Here's how the part is built. I have some questions about the finished solid (model axes, mm). A direction names the side the tool comes from. Coordinates: 2 decimals unless noted, no trailing zeros. Write each loop counter-clockwise with the first axis right and the second up, starting at its lowest first coordinate (ties: lowest second). Pieces come first, ordered by that corner, then holes.
Item 1: I want a section at B-B (y = -24). Please give me the cut outline in (x, z).
Item 2: I'm going to push flat-ended pins straight in: P1, Ø1.7, axis at y = 34, z = 107, coming from the +X side; P2, Ø1.8, axis at x = 4.5, y = 14, coming from the +Z side; P3, Ø1.8, axis at x = 4.5, z = 65.5, coming from the +Y side; P4, Ø3, axis at x = 3.5, y = -121.5, coming from the -Z side. Where does each tip first touch, or does it pass through?
Item 3: I want a section at C-C (x = 4). Count the separate pieces of the cut face and the enclosed holes in it, and give its area (3 significant figures).
Item 4: I want a section at A-A (z = -20.5). Please give me the cut outline in (x, y).
Item 5: For faces 1 (the face through (3, 59, 104)), 2 (the face through (3, 122, 80)), 3 (the face through (3, -59, -104)), which set-ups out of +Z, -Z, +X, -X, +Y, -Y let a thin tool reach every point of the face, with its end or its side?
Item 6: Please list where these lines run through material, in increasing order: line 1 (Y direction, x = 3.2, z = -45); line 2 (Y direction, x = 5.05, z = -76.5); line 3 (Z direction, x = 2.2, y = -13).
Item 7: If we mould it in two halves opening along Z, with no side actions, what happens to faces 4 (the face through (3, 125, -85)), 5 (the face through (3, -122, -80)), 6 (the face through (3, -104, 104))? For each: pulls with the +Z half, pulls with the -Z half, needs draft (parallel to the pull), parting line crosses it, or undercut.
from build123d import *

# Parameters (mm, degrees)
ESQUISSE1_W             = 208
ESQUISSE1_H             = 238
BOSS_EXTRU_1_DEPTH      = 6
ESQUISSE3_W             = 10
ESQUISSE3_H             = 6
ESQUISSE3_W_2           = 6
ESQUISSE3_H_2           = 10
BOSS_EXTRU_5_DEPTH      = 6
ESQUISSE4_R             = 1.4
ENL_V_MAT_EXTRU_1_DEPTH = 6


with BuildPart() as part:
    # Esquisse1 → Boss.-Extru.1 (new body)
    with BuildSketch(Plane(origin=(0, 0, 0), x_dir=(0, 0, -1), z_dir=(1, 0, 0))):
        Rectangle(ESQUISSE1_W, ESQUISSE1_H)
    extrude(amount=BOSS_EXTRU_1_DEPTH)

    # Esquisse3 → Boss.-Extru.5 (add)
    with BuildSketch(Plane(origin=(6, 0, 0), x_dir=(0, 0, -1), z_dir=(1, 0, 0))):
        with Locations((-85, -122)):
            Rectangle(ESQUISSE3_W, ESQUISSE3_H)
        with Locations((-45, -122)):
            Rectangle(ESQUISSE3_W, ESQUISSE3_H)
        with Locations((107, -34)):
            Rectangle(ESQUISSE3_W_2, ESQUISSE3_H_2)
        with Locations((-107, -84)):
            Rectangle(ESQUISSE3_W_2, ESQUISSE3_H_2)
        with Locations((-107, -34)):
            Rectangle(ESQUISSE3_W_2, ESQUISSE3_H_2)
        with Locations((107, -84)):
            Rectangle(ESQUISSE3_W_2, ESQUISSE3_H_2)
        with Locations((45, -122)):
            Rectangle(ESQUISSE3_W, ESQUISSE3_H)
        with Locations((85, -122)):
            Rectangle(ESQUISSE3_W, ESQUISSE3_H)
        with Locations((85, 122)):
            Rectangle(ESQUISSE3_W, ESQUISSE3_H)
        with Locations((45, 122)):
            Rectangle(ESQUISSE3_W, ESQUISSE3_H)
        with Locations((107, 84)):
            Rectangle(ESQUISSE3_W_2, ESQUISSE3_H_2)
        with Locations((107, 34)):
            Rectangle(ESQUISSE3_W_2, ESQUISSE3_H_2)
        with Locations((-107, 34)):
            Rectangle(ESQUISSE3_W_2, ESQUISSE3_H_2)
        with Locations((-107, 84)):
            Rectangle(ESQUISSE3_W_2, ESQUISSE3_H_2)
        with Locations((-45, 122)):
            Rectangle(ESQUISSE3_W, ESQUISSE3_H)
        with Locations((-85, 122)):
            Rectangle(ESQUISSE3_W, ESQUISSE3_H)
    extrude(amount=-BOSS_EXTRU_5_DEPTH)

    # Esquisse4 → Enlèv. mat.-Extru.1 (cut)
    with BuildSketch(Plane(origin=(6, 0, 0), x_dir=(0, 0, -1), z_dir=(1, 0, 0))):
        with Locations((-85, 122)):
            Circle(ESQUISSE4_R)
        with Locations((-45, 122)):
            Circle(ESQUISSE4_R)
        with Locations((-107, 84)):
            Circle(ESQUISSE4_R)
        with Locations((-107, 34)):
            Circle(ESQUISSE4_R)
        with Locations((107, 34)):
            Circle(ESQUISSE4_R)
        with Locations((107, 84)):
            Circle(ESQUISSE4_R)
        with Locations((45, 122)):
            Circle(ESQUISSE4_R)
        with Locations((85, 122)):
            Circle(ESQUISSE4_R)
        with Locations((85, -122)):
            Circle(ESQUISSE4_R)
        with Locations((45, -122)):
            Circle(ESQUISSE4_R)
        with Locations((107, -84)):
            Circle(ESQUISSE4_R)
        with Locations((107, -34)):
            Circle(ESQUISSE4_R)
        with Locations((-107, -34)):
            Circle(ESQUISSE4_R)
        with Locations((-107, -84)):
            Circle(ESQUISSE4_R)
        with Locations((-45, -122)):
            Circle(ESQUISSE4_R)
        with Locations((-85, -122)):
            Circle(ESQUISSE4_R)
    extrude(amount=-ENL_V_MAT_EXTRU_1_DEPTH, mode=Mode.SUBTRACT)


solid = part.part
Answer:
1. outline: (0, -104) - (6, -104) - (6, 104) - (0, 104) - close
2. P1: passes through
2. P2: stops at z = 104
2. P3: stops at y = 119
2. P4: stops at z = -90
3. separate pieces: 1
3. enclosed holes: 16
3. area: 50,400 mm2
4. outline: (0, -119) - (6, -119) - (6, 119) - (0, 119) - close
5. face 1: +Z, +X, -X
5. face 2: +X, -X, +Y
5. face 3: -Z, +X, -X
6. line 1: y = -125 to -123.4, -120.6 to 120.6, 123.4 to 125
6. line 2: y = -119 to 119
6. line 3: z = -104 to 104
7. face 4: needs draft
7. face 5: undercut
7. face 6: pulls with the +Z half
